Here's the drawing with two shaded views (mm, measured from the low corner). I have some questions. Round coordinates to 2 decimals unless told otherwise and drop trailing zeros. Order: outer loops, then holes, each group sorted by start corner. A loop starts at its lowest first (then second) coordinate and runs counter-clockwise, first axis right, second up.
Q1. If we section it at B-B (z = 38): Please give me the cut outline in (x, y), plus the area to 3 significant figures.
Q2. If I drill on line 1 (X direction, y = 17.5, z = 22); line 2 (X direction, y = 4, z = 25); line 3 (X direction, y = 12, z = 6), over which ranges is the centre line in solid material (lowest first)?
Q3. Will these pins go through, and if not, where does the flat tip stop? P1, Ø18.5, axis at x = 50, z = 25, coming from the +Y side; P2, Ø12, axis at x = 28.5, z = 28, coming from the +Y side; P3, Ø8, axis at y = 17.5, z = 44.5, coming from the -X side; P4, Ø8.5, axis at x = 80, y = 12.5, coming from the +Z side.
Q4. If we section it at A-A (x = 20): Please give me the cut outline in (y, z).
Q5. If we section it at D-D (x = 50): Please give me the cut outline in (y, z), plus the area to 3 significant figures.
Q6. We'd pull the mould along X, two halves only. Please class the marked faces 1, 2 and 3: pulls with the +X half, pulls with the -X half, needs draft (parallel to the pull), parting line crosses it, or undercut.
Q7. If we section it at C-C (y = 12.5): Please give me the cut outline in (x, z).
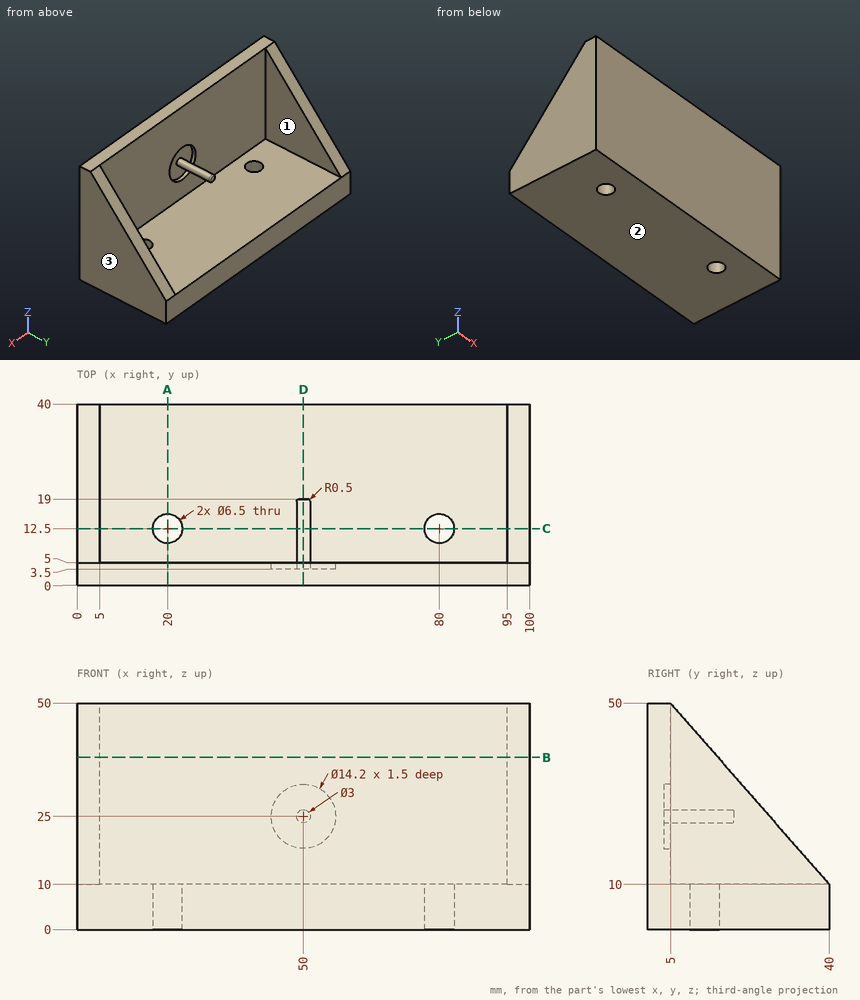
Solution:
1. outline: (0, 0) - (100, 0) - (100, 15.5) - (95, 15.5) - (95, 5) - (5, 5) - (5, 15.5) - (0, 15.5) - close
1. area: 605 mm2
2. line 1: x = 0 to 5, 95 to 100
2. line 2: x = 0 to 42.9, 48.5 to 51.5, 57.1 to 100
2. line 3: x = 0 to 16.79, 23.21 to 76.79, 83.21 to 100
3. P1: stops at y = 19
3. P2: stops at y = 5
3. P3: passes through
3. P4: stops at z = 10
4. outline: (0, 0) - (9.25, 0) - (9.25, 10) - (5, 10) - (5, 50) - (0, 50) - close; (15.75, 0) - (40, 0) - (40, 10) - (15.75, 10) - close
5. outline: (0, 0) - (40, 0) - (40, 10) - (5, 10) - (5, 17.9) - (3.5, 17.9) - (3.5, 23.5) - (18.5, 23.5) arc R0.5 ccw to (19, 24) - (19, 26) arc R0.5 ccw to (18.5, 26.5) - (3.5, 26.5) - (3.5, 32.1) - (5, 32.1) - (5, 50) - (0, 50) - close
5. area: 625 mm2
6. face 1: undercut
6. face 2: needs draft
6. face 3: pulls with the +X half
7. outline: (0, 0) - (16.75, 0) - (16.75, 10) - (5, 10) - (5, 41.43) - (0, 41.43) - close; (23.25, 0) - (76.75, 0) - (76.75, 10) - (23.25, 10) - close; circle Ø3 at (50, 25); (83.25, 0) - (100, 0) - (100, 41.43) - (95, 41.43) - (95, 10) - (83.25, 10) - close
